For this review, use the dimensioned drawing (mm, ordinates from the lowest corner) and the shaded views. Round coordinates to 2 decimals unless told otherwise and drop trailing zeros. Write each loop counter-clockwise with the first axis right and the second up, starting at its lowest first coordinate (ties: lowest second). Pieces come first, ordered by that corner, then holes. Notation, with made-up numbers: M 7.5,1.25 L 24.5,1.25 A18 cw 24.5,13.25 Z; hole C 18.5,-3 d9. An arc over 180 degrees is marked long. One line per question, with ' | ' between items. Start each with the question number.
Item 1: Add section B-B, the plane y = 7.25. State the section outline as (x, z) points.
Item 2: Add section C-C, the plane x = 6.5. State the section outline as (y, z) points.
Item 3: Add section D-D, the plane x = 8.75. State the section outline as (y, z) points (1 decimal).
Item 4: Insertion check: pin 1 Ø5 at (x, z) = (7, 5) entering from -Y; pin 2 Ø5 at (x, y) = (8, 7.5) entering from +Z; pin 3 Ø2 at (x, y) = (4.5, 2) entering from -Z; pin 4 Ø3.5 at (x, z) = (5, 5.77) entering from -Y. Each pin has a flat end and moves straight along its axis. Give the tip position at first contact, or say it passes through.
Item 5: Draft analysis for pull direction Z (two halves, no side actions). For the marked faces 1 and 2, state which applies: released by +Z, released by -Z, zero draft, split by the parting line, or undercut.
Item 6: Add section A-A, the plane z = 6.75. State the section outline as (x, y) points.
Item 7: For L1, parallel to X at y = 4, z = 4.5; L2, parallel to Z at x = 6.25, y = 3.5 (1 decimal); L3, parallel to Z at x = 4, y = 6.5 (1 decimal), list the stretches that pass through material, from the lowest coordinate up.
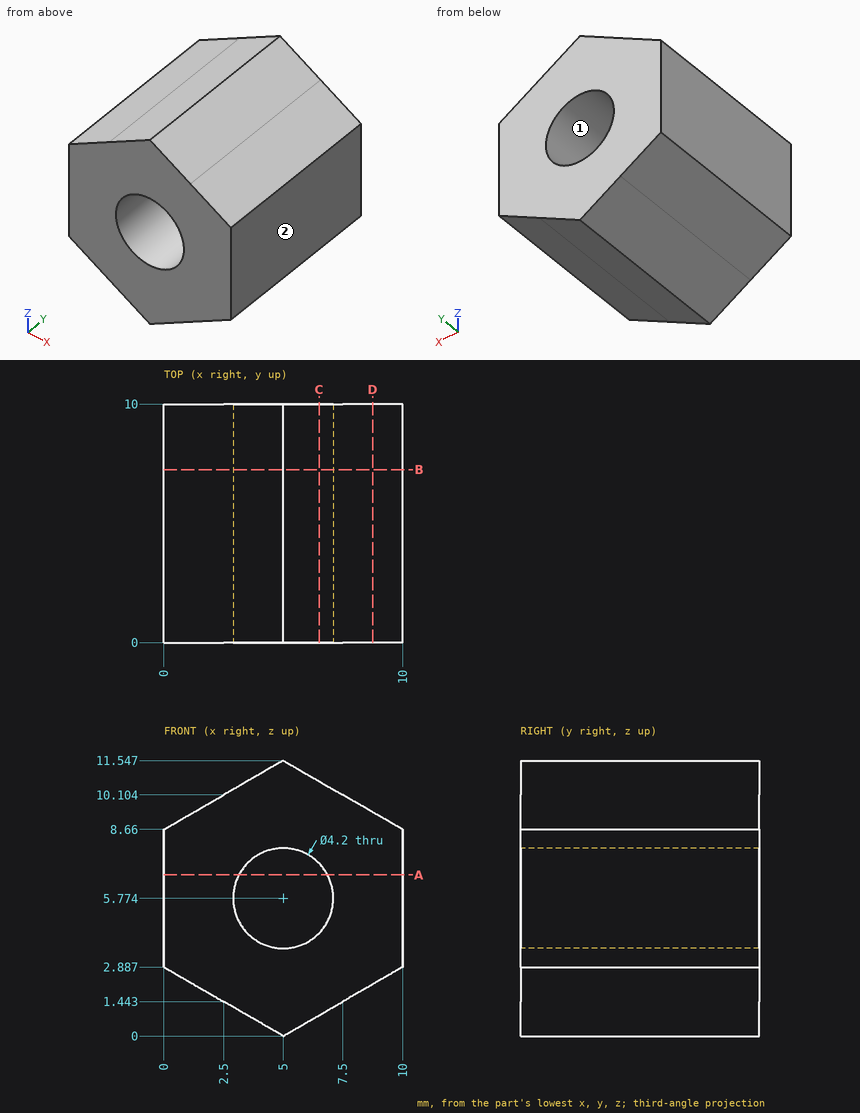
Computed values:
1) outline: M 0,2.89 L 2.5,1.44 L 5,0 L 7.5,1.44 L 10,2.89 L 10,8.66 L 7.5,10.1 L 5,11.55 L 2.5,10.1 L 0,8.66 Z; hole C 5,5.77 d4.2
2) outline: M 0,0.87 L 10,0.87 L 10,4.3 L 0,4.3 Z; M 0,7.24 L 10,7.24 L 10,10.68 L 0,10.68 Z
3) outline: M 0,2.2 L 10,2.2 L 10,9.4 L 0,9.4 Z
4) pin 1: stops at y = 0 | pin 2: stops at z = 11.26 | pin 3: stops at z = 0 | pin 4: passes through
5) face 1: undercut | face 2: zero draft
6) outline: M 0,0 L 3.14,0 L 3.14,10 L 0,10 Z; M 6.86,0 L 10,0 L 10,10 L 6.86,10 Z
7) L1: x = 0 to 3.33, 6.67 to 10 | L2: z = 0.7 to 4.1, 7.5 to 10.8 | L3: z = 0.6 to 3.9, 7.6 to 11
